Input: part model. Units: mm. Frame: model coordinates. A direction names the side the tool comes from. Round coordinates to 2 decimals unless told otherwise and drop trailing zeros. Loops run counter-clockwise (first coordinate to the right, second up) from the corner with the lowest first, then second, coordinate; pieces in that order, holes last. Notation, with made-up numbers: (22, -22.5) - (33, -22.5) arc R31 ccw to (33, 14.5) - close; hole circle Ø11 at (23.25, -28). An arc over 180 degrees is marked (long way). Write each question's results on one line, items separated by ' | '.
from build123d import *

# Parameters (mm, degrees)
SWEEP1_PROFILE_R = 1.5


with BuildPart() as part:
    # Esquisse1 → Révolution4 (revolve)
    with BuildSketch(Plane.XY):
        with BuildLine():
            Line((0, 5), (0, 6))
            ThreePointArc((0, 6), (5.684108375, 1.921174635), (3.640054945, -4.769696007))
            Line((3.640054945, -4.769696007), (3.640054945, -9.769696007))
            Line((3.640054945, -9.769696007), (0.5, -9.769696007))
            Line((0.5, -9.769696007), (0.5, -14.283094956))
            Line((0.5, -14.283094956), (0, -14.283094956))
            Line((0, -14.283094956), (0, -4.769696007))
            Line((0, -4.769696007), (1.5, -4.769696007))
            ThreePointArc((1.5, -4.769696007), (4.942088629, 0.758788496), (0, 5))
        make_face()
    revolve(axis=Axis((0, 0, 0), (0, 1, 0)))

    # Sweep1: sweep along a path in Sketch1
    with BuildLine(Plane.XY) as sweep1_path:
        Line((9.49641969, -2.980934088), (8.595599399, -4.835775301))
        Line((8.595599399, -4.835775301), (5.744918771, -6.566545682))
        Line((5.744918771, -6.566545682), (3.118220193, -7.177405817))
        Line((3.118220193, -7.177405817), (-3.118220193, -7.177405817))
        Line((-3.118220193, -7.177405817), (-5.744918771, -6.566545682))
        Line((-5.744918771, -6.566545682), (-8.595599399, -4.835775301))
        Line((-8.595599399, -4.835775301), (-9.49641969, -2.980934088))
    # Sweep1 profile (on start of the path) → Sweep1 (sweep)
    with BuildSketch(Plane(origin=(9.49641969, -2.980934088, 0), x_dir=(-0.8995277091216457, 0.4368637093217566, 0), z_dir=(-0.4368637093217566, -0.8995277091216457, 0))):
        Circle(SWEEP1_PROFILE_R)
    sweep(path=sweep1_path.line, transition=Transition.RIGHT)


solid = part.part
1. Mould query, pull axis X, two halves, no side actions, for faces 1 (the cylindrical face through (-10.427, -4.496, -0.066)), 2 (the flat face through (9.515, -2.99, -0.021)), 3 (the flat face through (0, -9.77, 1)). Classes: pulls with the +X half, pulls with the -X half, needs draft (parallel to the pull), parting line crosses it, or undercut.
Answer:
face 1: undercut | face 2: pulls with the +X half | face 3: needs draft
2. Section query C-C, the plane z = 0. Output: boundary loops of the cut face in (x, y), plus the area to 3 significant figures.
Answer:
outline: (-10.85, -3.64) - (-9.75, -5.89) - (-6.32, -7.97) - (-3.64, -8.6) - (-3.64, -9.77) - (-0.5, -9.77) - (-0.5, -14.28) - (0.5, -14.28) - (0.5, -9.77) - (3.64, -9.77) - (3.64, -8.6) - (6.32, -7.97) - (9.75, -5.89) - (10.85, -3.64) - (8.15, -2.33) - (7.44, -3.78) - (5.17, -5.16) - (3.64, -5.52) - (3.64, -4.77) arc R6 ccw (long way) to (-3.64, -4.77) - (-3.64, -5.52) - (-5.17, -5.16) - (-7.44, -3.78) - (-8.15, -2.33) - close; hole (-1.5, -4.77) - (1.5, -4.77) arc R5 ccw (long way) to start | area: 115 mm^2
3. Section query D-D, the plane x = 2.75. Output: boundary loops of the cut face in (y, z), plus the area to 3 significant figures.
Answer:
outline: (-9.77, -2.38) - (-4.77, -2.38) arc R5.33 ccw (long way) to (-4.77, 2.38) - (-9.77, 2.38) - close; hole circle Ø8.35 at (0, 0) | area: 56.6 mm^2
4. Contact query for flat-ended pins moving along their axis: pin 1 (1 mm diameter, centred on y = -3.5, z = 3, fed in from +X); pin 2 (5 mm diameter, centred on x = 5.5, y = -2.5, fed in from -Z); pin 3 (5 mm diameter, centred on x = -6.5, y = 0.5, fed in from +Z). Output: stop coordinate, or through.
Answer:
pin 1: x = 4.37 | pin 2: z = -4.84 | pin 3: z = 4.45
5. Section query A-A, the plane x = 0. Output: boundary loops of the cut face in (y, z).
Answer:
outline: (-14.28, -0.5) - (-9.77, -0.5) - (-9.77, -3.64) - (-4.77, -3.64) arc R6 ccw (long way) to (-4.77, 3.64) - (-9.77, 3.64) - (-9.77, 0.5) - (-14.28, 0.5) - close; hole (-4.77, -1.5) arc R5 ccw (long way) to (-4.77, 1.5) - close
6. Set-up query: faces 4 (the flat face through (0, -14.283, 0)), 5 (the cylindrical face through (-0.108, -12.058, 0.488)), 6 (the flat face through (0, -4.77, 0)). Return all of +Z, -Z, +X, -X, +Y, -Y with unobstructed straight access to the full face (end or side cutting, diameter ignored); none if empty.
Answer:
face 4: +Z, -Z, +X, -X, -Y | face 5: -Y | face 6: none
7. Line query: line 1 (X direction, y = -2.75, z = 0.75); line 2 (X direction, y = -1.75, z = 1); line 3 (Y direction, x = 3, z = 0.5). Output: solid intervals per line, ascending. Write a range as [from, to].
Answer:
line 1: [-9.02, -8.16], [-5.28, -4.11], [4.11, 5.28], [8.16, 9.02] | line 2: [-5.65, -4.58], [4.58, 5.65] | line 3: [-9.77, -3.97], [3.97, 5.17]
8. Section query B-B, the plane z = -3. Output: boundary loops of the cut face in (x, y).
Answer:
outline: (-2.06, -9.77) - (2.06, -9.77) - (2.06, -4.77) arc R5.2 ccw (long way) to (-2.06, -4.77) - close; hole circle Ø8 at (0, 0)
